Read the model definition and answer for the solid it produces. Units are mm, in the model's axes. Round coordinates to 2 decimals unless told otherwise and drop trailing zeros. Write each loop counter-clockwise with the first axis right and the second up, starting at its lowest first coordinate (ties: lowest second). Pieces come first, ordered by that corner, then holes. Notation, with made-up numbers: (33, 7) -> (59, 7) arc R7 ccw to (59, 20) -> close; hole circle Ø3 at (-29.5, 69.5). An arc over 180 degrees is marked (long way). Return JSON: item names as keys, results as strings. Group by question number.
(1) A cutting plane is placed at B-B on x = 9. Give the vertices of the cut face in (y, z) (3 decimals), then the cut area to 3 significant figures.
(2) A cutting plane is placed at C-C on z = 3. Give the vertices of the cut face in (x, y) (1 decimal), then the cut area to 3 significant figures.
(3) A cutting plane is placed at D-D on y = 23.5. Give the vertices of the cut face in (x, z) (3 decimals), then the cut area to 3 significant figures.
(4) A cutting plane is placed at A-A on y = 6.35. Give the vertices of the cut face in (x, z) (3 decimals), then the cut area to 3 significant figures.
(5) The mould has two halves that part along Z. Classify faces 1 (the flat face through (20, 28.575, 9)), 2 (the flat face through (19, 14, 19.05)), 3 (the cylindrical face through (19.639, 9.498, 9.938)): released by +Z, released by -Z, zero draft, split by the parting line, or undercut.
(6) Given pin 1 (5.5 mm diameter, centred on x = 19.37, y = 21.43, fed in from +Z); pin 2 (6 mm diameter, centred on x = 33.5, z = 9, fed in from -Y), each flat-ended and moving along its own axis, determine where each tip first touches the part or whether it passes through.
(7) Straight lines are drawn through the part: line 1 (Y direction, x = 22.5, z = 10.25) (3 decimals); line 2 (Z direction, x = 25, y = 9.25); line 3 (Z direction, x = 22, y = 6.35). For each, find the intervals that lie inside material, in ascending order.
Autodesk Inventor part; units mm, degrees
ref_plane "YZ Plane" through (0, 0, 0) normal (1, 0, 0) x (0, 1, 0)
ref_plane "XZ Plane" through (0, 0, 0) normal (0, 1, 0) x (-1, 0, 0)
ref_plane "XY Plane" through (0, 0, 0) normal (0, 0, 1) x (1, 0, 0)
sketch "Sketch1" plane through (0, 0, 0) normal (0, 0, 1) x (1, 0, 0)
  line L0 (0, 0) -> (38.735, 0)
  line L1 (38.735, 0) -> (38.735, 28.575)
  line L2 (38.735, 28.575) -> (0, 28.575)
  line L3 (0, 28.575) -> (0, 0)
  dimension "d0" = 38.735
  dimension "d1" = 28.575
extrude "Extrusion1" add sketch "Sketch1" along normal blind 19.05
sketch "Sketch2" plane through (38.735, 0, 0) normal (1, 0, 0) x (0, 0, -1)
  line L0 (0, 0) -> (-19.05, 0)
  line L1 (0, 0) -> (-19.05, 0)
  line L2 (-19.05, 0) -> (-9.525, 0)
  line L3 (-9.525, 0) -> (-9.525, 28.575)
  line L4 (0, 28.575) -> (-19.05, 28.575)
  line L5 (-9.525, 0) -> (-9.525, 12.7)
  line L6 (-9.525, 12.7) -> (-9.525, 6.35)
  circle A0 centre (-9.525, 6.35) radius 3.175
  dimension "d4" = 12.7
  dimension "d5" = 6.35
  dimension "d6" = 6.35
extrude "Extrusion2" cut sketch "Sketch2" against normal blind 76.2
sketch "Sketch3" plane through (0, 0, 19.05) normal (0, 0, 1) x (1, 0, 0)
  line L0 (0, 0) -> (0, 28.575)
  line L1 (0, 28.575) -> (0, 0)
  line L2 (0, 28.575) -> (38.735, 28.575)
  line L3 (38.735, 28.575) -> (19.3675, 28.575)
  line L4 (19.3675, 28.575) -> (19.3675, 0)
  line L5 (19.3675, 0) -> (19.3675, 14.2875)
  line L6 (19.3675, 14.2875) -> (19.3675, 28.575)
  line L7 (19.3675, 28.575) -> (19.3675, 21.4312)
  circle A0 centre (19.3675, 21.4312) radius 4.7625
  dimension "d9" = 9.525
extrude "Extrusion3" cut sketch "Sketch3" against normal blind 76.2
thread "Thread1"
properties part number "coupler"
Checks:
{
 "1": {"outline": "(0, 0) -> (28.575, 0) -> (28.575, 19.05) -> (0, 19.05) -> close; hole circle Ø6.35 at (6.35, 9.525)", "area": "513 mm^2"},
 "2": {"outline": "(0, 0) -> (38.7, 0) -> (38.7, 28.6) -> (0, 28.6) -> close; hole circle Ø9.5 at (19.4, 21.4)", "area": "1,040 mm^2"},
 "3": {"outline": "(0, 0) -> (15.078, 0) -> (15.078, 19.05) -> (0, 19.05) -> close; (23.657, 0) -> (38.735, 0) -> (38.735, 19.05) -> (23.657, 19.05) -> close", "area": "574 mm^2"},
 "4": {"outline": "(0, 0) -> (38.735, 0) -> (38.735, 6.35) -> (0, 6.35) -> close; (0, 12.7) -> (38.735, 12.7) -> (38.735, 19.05) -> (0, 19.05) -> close", "area": "492 mm^2"},
 "5": {"face 1": "zero draft", "face 2": "released by +Z", "face 3": "undercut"},
 "6": {"pin 1": "passes through", "pin 2": "stops at y = 0"},
 "7": {"line 1": "y = 0 to 3.259, 9.441 to 17.844, 25.019 to 28.575", "line 2": "z = 0 to 8.23, 10.82 to 19.05", "line 3": "z = 0 to 6.35, 12.7 to 19.05"}
}
